Part model, mm, in its own coordinate system. A direction names the side the tool comes from. Round coordinates to 2 decimals unless told otherwise and drop trailing zeros. Loops run counter-clockwise (first coordinate to the right, second up) from the corner with the lowest first, then second, coordinate; pieces in that order, holes last.
1) Band-saw the part on B-B, the plane z = -95. Write the cut outline in (x, y), then the cut area to 3 significant figures.
2) Band-saw the part on A-A, the plane x = 228.5. Write the cut outline in (y, z), then the cut area to 4 significant figures.
3) Mould opens along Z. For faces 3 (the flat face through (4.44, 2.28, -230.92)), 4 (the flat face through (236, 0, -41)), 5 (the cylindrical face through (179.01, 2.28, -59.28)) say: +Z half, -Z half, draft (parallel to the pull), parting line (faces both ways), or undercut.
4) Drop flat-ended pins along their axis: P1, Ø2, axis at y = 1.5, z = -231, coming from the +X side; P2, Ø1.3, axis at y = 3, z = -232, coming from the +X side. Give the stop position or say it passes through.
5) Probe line 1 (X direction, y = 1.05, z = -22.5); line 2 (X direction, y = 2.95, z = -214); line 3 (Z direction, x = 459.5, y = 3.5). List the from-to ranges inside material, lowest first.
6) 3-axis set-ups, long thin cutter, end or side, ignore diameter. For faces 1 (the cylindrical face through (299.99, 2.28, -180.72)), 2 (the flat face through (236, 4.5, -41)): which of +Z, -Z, +X, -X, +Y, -Y reach the whole face in a straight line?
7) Band-saw the part on C-C, the plane y = 3.65. State how many separate pieces and enclosed holes the cut face has, then the cut area to 3 significant figures.
from build123d import *

# Parameters (mm, degrees)
SKETCH_1_W          = 479
SKETCH_1_H          = 237
EXTRUDE_1_DEPTH     = 4.5
CUT_EXTRUDE_1_REACH = 536.444
SKETCH_2_R          = 2
SKETCH_2_W          = 41
SKETCH_2_H          = 8.5
CUT_EXTRUDE_2_DEPTH = 10


with BuildPart() as part:
    # 草图1 → 凸台-拉伸1 (new body)
    with BuildSketch(Plane(origin=(0, 0, 0), x_dir=(1, 0, 0), z_dir=(0, 1, 0))):
        with Locations((239.5, 118.5)):
            Rectangle(SKETCH_1_W, SKETCH_1_H)
    extrude(amount=EXTRUDE_1_DEPTH)

    # 草图2 → 切除-拉伸1 (cut, up to next)
    with BuildSketch(Plane(origin=(0, 4.5, 0), x_dir=(1, 0, 0), z_dir=(0, 1, 0)), mode=Mode.PRIVATE) as cut_extrude_1_sk1:
        with Locations(Location((399, 22.5, 0), (0, 0, 270))):
            Circle(SKETCH_2_R)
    cut_extrude_1_tool1 = extrude(cut_extrude_1_sk1.sketch, amount=-CUT_EXTRUDE_1_REACH, mode=Mode.PRIVATE) & part.part
    # 草图2 → 切除-拉伸1 (cut, up to next)
    with BuildSketch(Plane(origin=(0, 4.5, 0), x_dir=(1, 0, 0), z_dir=(0, 1, 0)), mode=Mode.PRIVATE) as cut_extrude_1_sk2:
        with Locations(Location((375, 22.5, 0), (0, 0, 270))):
            Circle(SKETCH_2_R)
    cut_extrude_1_tool2 = extrude(cut_extrude_1_sk2.sketch, amount=-CUT_EXTRUDE_1_REACH, mode=Mode.PRIVATE) & part.part
    # 草图2 → 切除-拉伸1 (cut, up to next)
    with BuildSketch(Plane(origin=(0, 4.5, 0), x_dir=(1, 0, 0), z_dir=(0, 1, 0)), mode=Mode.PRIVATE) as cut_extrude_1_sk3:
        with Locations(Location((104, 22.5, 0), (0, 0, 90))):
            Circle(SKETCH_2_R)
    cut_extrude_1_tool3 = extrude(cut_extrude_1_sk3.sketch, amount=-CUT_EXTRUDE_1_REACH, mode=Mode.PRIVATE) & part.part
    # 草图2 → 切除-拉伸1 (cut, up to next)
    with BuildSketch(Plane(origin=(0, 4.5, 0), x_dir=(1, 0, 0), z_dir=(0, 1, 0)), mode=Mode.PRIVATE) as cut_extrude_1_sk4:
        with Locations(Location((80, 22.5, 0), (0, 0, 90))):
            Circle(SKETCH_2_R)
    cut_extrude_1_tool4 = extrude(cut_extrude_1_sk4.sketch, amount=-CUT_EXTRUDE_1_REACH, mode=Mode.PRIVATE) & part.part
    # 草图2 → 切除-拉伸1 (cut, up to next)
    with BuildSketch(Plane(origin=(0, 4.5, 0), x_dir=(1, 0, 0), z_dir=(0, 1, 0)), mode=Mode.PRIVATE) as cut_extrude_1_sk5:
        with Locations(Location((459.5, 193.9, 0), (0, 0, 270))):
            Circle(SKETCH_2_R)
    cut_extrude_1_tool5 = extrude(cut_extrude_1_sk5.sketch, amount=-CUT_EXTRUDE_1_REACH, mode=Mode.PRIVATE) & part.part
    # 草图2 → 切除-拉伸1 (cut, up to next)
    with BuildSketch(Plane(origin=(0, 4.5, 0), x_dir=(1, 0, 0), z_dir=(0, 1, 0)), mode=Mode.PRIVATE) as cut_extrude_1_sk6:
        with Locations(Location((459.5, 169.9, 0), (0, 0, 270))):
            Circle(SKETCH_2_R)
    cut_extrude_1_tool6 = extrude(cut_extrude_1_sk6.sketch, amount=-CUT_EXTRUDE_1_REACH, mode=Mode.PRIVATE) & part.part
    # 草图2 → 切除-拉伸1 (cut, up to next)
    with BuildSketch(Plane(origin=(0, 4.5, 0), x_dir=(1, 0, 0), z_dir=(0, 1, 0)), mode=Mode.PRIVATE) as cut_extrude_1_sk7:
        with Locations(Location((19.5, 169.9, 0), (0, 0, 90))):
            Circle(SKETCH_2_R)
    cut_extrude_1_tool7 = extrude(cut_extrude_1_sk7.sketch, amount=-CUT_EXTRUDE_1_REACH, mode=Mode.PRIVATE) & part.part
    # 草图2 → 切除-拉伸1 (cut, up to next)
    with BuildSketch(Plane(origin=(0, 4.5, 0), x_dir=(1, 0, 0), z_dir=(0, 1, 0)), mode=Mode.PRIVATE) as cut_extrude_1_sk8:
        with Locations(Location((19.5, 193.9, 0), (0, 0, 90))):
            Circle(SKETCH_2_R)
    cut_extrude_1_tool8 = extrude(cut_extrude_1_sk8.sketch, amount=-CUT_EXTRUDE_1_REACH, mode=Mode.PRIVATE) & part.part
    # 草图2 → 切除-拉伸1 (cut, up to next)
    with BuildSketch(Plane(origin=(0, 4.5, 0), x_dir=(1, 0, 0), z_dir=(0, 1, 0)), mode=Mode.PRIVATE) as cut_extrude_1_sk9:
        with Locations(Location((94.5, 214, 0), (0, 0, 270))):
            Circle(SKETCH_2_R)
    cut_extrude_1_tool9 = extrude(cut_extrude_1_sk9.sketch, amount=-CUT_EXTRUDE_1_REACH, mode=Mode.PRIVATE) & part.part
    # 草图2 → 切除-拉伸1 (cut, up to next)
    with BuildSketch(Plane(origin=(0, 4.5, 0), x_dir=(1, 0, 0), z_dir=(0, 1, 0)), mode=Mode.PRIVATE) as cut_extrude_1_sk10:
        with Locations(Location((114.5, 214, 0), (0, 0, 270))):
            Circle(SKETCH_2_R)
    cut_extrude_1_tool10 = extrude(cut_extrude_1_sk10.sketch, amount=-CUT_EXTRUDE_1_REACH, mode=Mode.PRIVATE) & part.part
    # 草图2 → 切除-拉伸1 (cut, up to next)
    with BuildSketch(Plane(origin=(0, 4.5, 0), x_dir=(1, 0, 0), z_dir=(0, 1, 0)), mode=Mode.PRIVATE) as cut_extrude_1_sk11:
        with Locations(Location((364.5, 214, 0), (0, 0, 90))):
            Circle(SKETCH_2_R)
    cut_extrude_1_tool11 = extrude(cut_extrude_1_sk11.sketch, amount=-CUT_EXTRUDE_1_REACH, mode=Mode.PRIVATE) & part.part
    # 草图2 → 切除-拉伸1 (cut, up to next)
    with BuildSketch(Plane(origin=(0, 4.5, 0), x_dir=(1, 0, 0), z_dir=(0, 1, 0)), mode=Mode.PRIVATE) as cut_extrude_1_sk12:
        with Locations(Location((384.5, 214, 0), (0, 0, 90))):
            Circle(SKETCH_2_R)
    cut_extrude_1_tool12 = extrude(cut_extrude_1_sk12.sketch, amount=-CUT_EXTRUDE_1_REACH, mode=Mode.PRIVATE) & part.part
    # 草图2 → 切除-拉伸1 (cut, up to next)
    with BuildSketch(Plane(origin=(0, 4.5, 0), x_dir=(1, 0, 0), z_dir=(0, 1, 0)), mode=Mode.PRIVATE) as cut_extrude_1_sk13:
        Polygon((0, 237), (0, 225), (9, 237), align=None)
    cut_extrude_1_tool13 = extrude(cut_extrude_1_sk13.sketch, amount=-CUT_EXTRUDE_1_REACH, mode=Mode.PRIVATE) & part.part
    # 草图2 → 切除-拉伸1 (cut, up to next)
    with BuildSketch(Plane(origin=(0, 4.5, 0), x_dir=(1, 0, 0), z_dir=(0, 1, 0)), mode=Mode.PRIVATE) as cut_extrude_1_sk14:
        Polygon((470, 237), (479, 237), (479, 225), align=None)
    cut_extrude_1_tool14 = extrude(cut_extrude_1_sk14.sketch, amount=-CUT_EXTRUDE_1_REACH, mode=Mode.PRIVATE) & part.part
    # 草图2 → 切除-拉伸1 (cut, up to next)
    with BuildSketch(Plane(origin=(0, 4.5, 0), x_dir=(1, 0, 0), z_dir=(0, 1, 0)), mode=Mode.PRIVATE) as cut_extrude_1_sk15:
        with Locations((104.5, 232.75)):
            Rectangle(SKETCH_2_W, SKETCH_2_H)
    cut_extrude_1_tool15 = extrude(cut_extrude_1_sk15.sketch, amount=-CUT_EXTRUDE_1_REACH, mode=Mode.PRIVATE) & part.part
    # 草图2 → 切除-拉伸1 (cut, up to next)
    with BuildSketch(Plane(origin=(0, 4.5, 0), x_dir=(1, 0, 0), z_dir=(0, 1, 0)), mode=Mode.PRIVATE) as cut_extrude_1_sk16:
        with Locations((374.5, 232.75)):
            Rectangle(SKETCH_2_W, SKETCH_2_H)
    cut_extrude_1_tool16 = extrude(cut_extrude_1_sk16.sketch, amount=-CUT_EXTRUDE_1_REACH, mode=Mode.PRIVATE) & part.part
    add(cut_extrude_1_tool1.solids().sort_by_distance((399, 4.5, -22.5))[0], mode=Mode.SUBTRACT)
    add(cut_extrude_1_tool2.solids().sort_by_distance((375, 4.5, -22.5))[0], mode=Mode.SUBTRACT)
    add(cut_extrude_1_tool3.solids().sort_by_distance((104, 4.5, -22.5))[0], mode=Mode.SUBTRACT)
    add(cut_extrude_1_tool4.solids().sort_by_distance((80, 4.5, -22.5))[0], mode=Mode.SUBTRACT)
    add(cut_extrude_1_tool5.solids().sort_by_distance((459.5, 4.5, -193.9))[0], mode=Mode.SUBTRACT)
    add(cut_extrude_1_tool6.solids().sort_by_distance((459.5, 4.5, -169.9))[0], mode=Mode.SUBTRACT)
    add(cut_extrude_1_tool7.solids().sort_by_distance((19.5, 4.5, -169.9))[0], mode=Mode.SUBTRACT)
    add(cut_extrude_1_tool8.solids().sort_by_distance((19.5, 4.5, -193.9))[0], mode=Mode.SUBTRACT)
    add(cut_extrude_1_tool9.solids().sort_by_distance((94.5, 4.5, -214))[0], mode=Mode.SUBTRACT)
    add(cut_extrude_1_tool10.solids().sort_by_distance((114.5, 4.5, -214))[0], mode=Mode.SUBTRACT)
    add(cut_extrude_1_tool11.solids().sort_by_distance((364.5, 4.5, -214))[0], mode=Mode.SUBTRACT)
    add(cut_extrude_1_tool12.solids().sort_by_distance((384.5, 4.5, -214))[0], mode=Mode.SUBTRACT)
    add(cut_extrude_1_tool13.solids().sort_by_distance((3, 4.5, -233))[0], mode=Mode.SUBTRACT)
    add(cut_extrude_1_tool14.solids().sort_by_distance((476, 4.5, -233))[0], mode=Mode.SUBTRACT)
    add(cut_extrude_1_tool15.solids().sort_by_distance((104.5, 4.5, -232.75))[0], mode=Mode.SUBTRACT)
    add(cut_extrude_1_tool16.solids().sort_by_distance((374.5, 4.5, -232.75))[0], mode=Mode.SUBTRACT)

    # 草图3 → 切除-拉伸2 (cut)
    with BuildSketch(Plane(origin=(0, 4.5, 0), x_dir=(1, 0, 0), z_dir=(0, 1, 0))):
        with BuildLine():
            Line((289.5, 55), (189.5, 55))
            ThreePointArc((189.5, 55), (178.893398282, 59.393398282), (174.5, 70))
            Line((174.5, 70), (174.5, 170))
            ThreePointArc((174.5, 170), (178.893398282, 180.606601718), (189.5, 185))
            Line((189.5, 185), (289.5, 185))
            ThreePointArc((289.5, 185), (300.106601718, 180.606601718), (304.5, 170))
            Line((304.5, 170), (304.5, 70))
            ThreePointArc((304.5, 70), (300.106601718, 59.393398282), (289.5, 55))
        make_face()
    extrude(amount=-CUT_EXTRUDE_2_DEPTH, mode=Mode.SUBTRACT)


solid = part.part
Reported:
1. outline: (0, 0) - (174.5, 0) - (174.5, 4.5) - (0, 4.5) - close; (304.5, 0) - (479, 0) - (479, 4.5) - (304.5, 4.5) - close
1. area: 1,570 mm2
2. outline: (0, -237) - (4.5, -237) - (4.5, -185) - (0, -185) - close; (0, -55) - (4.5, -55) - (4.5, 0) - (0, 0) - close
2. area: 481.5 mm2
3. face 3: -Z half
3. face 4: draft
3. face 5: undercut
4. P1: stops at x = 475.25
4. P2: stops at x = 474.24
5. line 1: x = 0 to 78, 82 to 102, 106 to 373, 377 to 397, 401 to 479
5. line 2: x = 0 to 92.5, 96.5 to 112.5, 116.5 to 362.5, 366.5 to 382.5, 386.5 to 479
5. line 3: z = -237 to -195.9, -191.9 to -171.9, -167.9 to 0
6. face 1: +Y, -Y
6. face 2: +Z, -Z, +X, -X, +Y
7. separate pieces: 1
7. enclosed holes: 13
7. area: 95,900 mm2
